from build123d import *

# Parameters (mm, degrees)
SKETCH_3_R               = 80
EXTRUDE_1_DEPTH          = 80
SKETCH_4_R               = 102.5
EXTRUDE_2_DEPTH          = 100
SKETCH_5_R               = 130
EXTRUDE_3_DEPTH          = 40
SKETCH_6_W               = 22
SKETCH_6_H               = 240.840734586
EXTRUDE_4_DEPTH          = 10
SHELL_START              = 82
SHELL_1_OUTLINE_R        = 100.5
SHELL_1_DEPTH            = 138
SHELL_START_2            = 2
SHELL_1_2_OUTLINE_R      = 78
SHELL_1_2_DEPTH          = 80
SHELL_START_3            = 182
SHELL_1_3_OUTLINE_R      = 128
SHELL_1_3_OUTLINE_R_2    = 100.5
SHELL_1_3_DEPTH          = 38
SHELL_START_4            = 212
SHELL_1_4_DEPTH          = 8
SKETCH_7_R               = 8.399329468
EXTRUDE_5_DEPTH          = 20
PATTERN_CIRCULAR_1_COUNT = 3
SKETCH_9_W               = 22
SKETCH_9_H               = 2
CUT_EXTRUDE_1_DEPTH      = 365.969552782
SKETCH_10_W              = 2
SKETCH_10_H              = 236.138085802
SKETCH_10_H_2            = 174.695606664
EXTRUDE_6_DEPTH          = 3
SKETCH_11_W              = 22
SKETCH_11_H              = 10
EXTRUDE_7_DEPTH          = 2
SKETCH_12_R              = 9.35670837
CUT_EXTRUDE_2_DEPTH      = 360.759328521
SKETCH_13_R              = 2.613319885
EXTRUDE_8_DEPTH          = 16
SKETCH_14_R              = 0.941183601
EXTRUDE_9_DEPTH          = 10


# Read off the part's stored shape, not the designer's step: 抽壳1
with BuildPart() as part:
    # 草图3 → 凸台-拉伸1 (new body)
    with BuildSketch(Plane(origin=(0, 0, 0), x_dir=(1, 0, 0), z_dir=(0, 1, 0))):
        with Locations(Location((0, 0, 0), (0, 0, 270))):
            Circle(SKETCH_3_R)
    extrude(amount=EXTRUDE_1_DEPTH)

    # 草图4 → 凸台-拉伸2 (add)
    with BuildSketch(Plane(origin=(0, 80, 0), x_dir=(1, 0, 0), z_dir=(0, 1, 0))):
        with Locations(Location((0, 0, 0), (0, 0, 270))):
            Circle(SKETCH_4_R)
    extrude(amount=EXTRUDE_2_DEPTH)

    # 草图5 → 凸台-拉伸3 (add)
    with BuildSketch(Plane(origin=(0, 180, 0), x_dir=(1, 0, 0), z_dir=(0, 1, 0))):
        with Locations(Location((0, 0, 0), (0, 0, 270))):
            Circle(SKETCH_5_R)
    extrude(amount=EXTRUDE_3_DEPTH)

    # 草图6 → 凸台-拉伸4 (add)
    with BuildSketch(Plane(origin=(0, 220, 0), x_dir=(1, 0, 0), z_dir=(0, 1, 0))):
        with Locations((117.8420905, -121.866187138)):
            Rectangle(SKETCH_6_W, SKETCH_6_H)
    extrude(amount=-EXTRUDE_4_DEPTH)

    # 抽壳1 outline → 抽壳1 (cut)
    with BuildSketch(Plane(origin=(0, 0, 0), x_dir=(1, 0, 0), z_dir=(0, 1, 0)).offset(SHELL_START)):
        Circle(SHELL_1_OUTLINE_R)
    extrude(amount=SHELL_1_DEPTH, mode=Mode.SUBTRACT)

    # Shell 1 2 outline → Shell 1 2 (cut)
    with BuildSketch(Plane(origin=(0, 0, 0), x_dir=(1, 0, 0), z_dir=(0, 1, 0)).offset(SHELL_START_2)):
        Circle(SHELL_1_2_OUTLINE_R)
    extrude(amount=SHELL_1_2_DEPTH, mode=Mode.SUBTRACT)

    # Shell 1 3 outline → Shell 1 3 (cut)
    with BuildSketch(Plane(origin=(0, 0, 0), x_dir=(1, 0, 0), z_dir=(0, 1, 0)).offset(SHELL_START_3)):
        Circle(SHELL_1_3_OUTLINE_R)
        Circle(SHELL_1_3_OUTLINE_R_2, mode=Mode.SUBTRACT)
    extrude(amount=SHELL_1_3_DEPTH, mode=Mode.SUBTRACT)

    # Shell 1 4 outline → Shell 1 4 (cut)
    with BuildSketch(Plane(origin=(0, 0, 0), x_dir=(1, 0, 0), z_dir=(0, 1, 0)).offset(SHELL_START_4)):
        with BuildLine():
            ThreePointArc((126.8420905, -17.178011456), (120.483699417, -43.216642337), (108.8420905, -67.360220721))
            Line((108.8420905, -67.360220721), (108.8420905, -240.286554431))
            Line((108.8420905, -240.286554431), (126.8420905, -240.286554431))
            Line((126.8420905, -240.286554431), (126.8420905, -17.178011456))
        make_face()
    extrude(amount=SHELL_1_4_DEPTH, mode=Mode.SUBTRACT)

    # 草图7 → 凸台-拉伸5 (add)
    with BuildSketch(Plane.XZ):
        with Locations(Location((0, 63.429571018, 0), (0, 0, 90))):
            Circle(SKETCH_7_R)
    extrude_5 = extrude(amount=EXTRUDE_5_DEPTH)

    # 阵列(圆周)1: 凸台-拉伸5 ×3 about axis
    pattern_circular_1_axis = Axis((0, 0, 0), (0, 1, 0))
    for i in range(1, PATTERN_CIRCULAR_1_COUNT):
        add(extrude_5.rotate(pattern_circular_1_axis, i * 360 / PATTERN_CIRCULAR_1_COUNT))

    # 草图9 → 切除-拉伸1 (cut, through all)
    with BuildSketch(Plane(origin=(0, 220, 0), x_dir=(1, 0, 0), z_dir=(0, 1, 0))):
        with Locations((117.8420905, -241.286554431)):
            Rectangle(SKETCH_9_W, SKETCH_9_H)
    extrude(amount=-CUT_EXTRUDE_1_DEPTH, mode=Mode.SUBTRACT)

    # 草图10 → 凸台-拉伸6 (add)
    with BuildSketch(Plane(origin=(0, 220, 0), x_dir=(1, 0, 0), z_dir=(0, 1, 0))):
        with Locations((109.8420905, -122.21751153)):
            Rectangle(SKETCH_10_W, SKETCH_10_H)
        with Locations((125.8420905, -152.938751099)):
            Rectangle(SKETCH_10_W, SKETCH_10_H_2)
    extrude(amount=-EXTRUDE_6_DEPTH)

    # 草图11 → 凸台-拉伸7 (add)
    with BuildSketch(Plane.XY.offset(240.286554431)):
        with Locations((117.8420905, 215)):
            Rectangle(SKETCH_11_W, SKETCH_11_H)
    extrude(amount=EXTRUDE_7_DEPTH)

    # 草图12 → 切除-拉伸2 (cut, through all)
    with BuildSketch(Plane(origin=(0, 212, 0), x_dir=(1, 0, 0), z_dir=(0, 1, 0))):
        with Locations(Location((117.8420905, -231.286554431, 0), (0, 0, 254.128345291))):
            Circle(SKETCH_12_R)
    extrude(amount=-CUT_EXTRUDE_2_DEPTH, mode=Mode.SUBTRACT)

    # 草图13 → 凸台-拉伸8 (add)
    with BuildSketch(Plane(origin=(128.8420905, 0, 0), x_dir=(0, 0, -1), z_dir=(1, 0, 0))):
        with Locations((-232.319143826, 214.997371462)):
            Circle(SKETCH_13_R)
    extrude(amount=EXTRUDE_8_DEPTH)

    # 草图14 → 凸台-拉伸9 (add)
    with BuildSketch(Plane(origin=(144.8420905, 0, 0), x_dir=(0, 0, -1), z_dir=(1, 0, 0))):
        with Locations((-232.319143826, 214.997371462)):
            Circle(SKETCH_14_R)
    extrude(amount=EXTRUDE_9_DEPTH)


solid = part.part
CAD build for the part. Positions are in the model's coordinates, mm. A direction names the side the tool comes from. Round coordinates to 2 decimals unless told otherwise and drop trailing zeros. Write each loop counter-clockwise with the first axis right and the second up, starting at its lowest first coordinate (ties: lowest second). Pieces come first, ordered by that corner, then holes.
(1) Slice it at D-D, the plane z = -50. Write the cut outline in (x, y), and give its area (3 significant figures).
(2) Slice it at A-A, the plane z = 153.5. Write the cut outline in (x, y).
(3) Probe line 1 along X through (y, z) = (210, 0); line 2 along X through (y, z) = (25, 0). List the from-to ranges inside material, lowest first.
(4) Slice it at C-C, the plane y = 26. Write the cut outline in (x, z).
(5) 3-axis set-ups, long thin cutter, end or side, ignore diameter. For faces 1 (the face through (118, 216, 240.287)), 2 (the face through (-10.154, 41.44, -77.336)), 3 (the face through (118, 210, 128)), 4 (the face through (39, 180, 96)): which of +Z, -Z, +X, -X, +Y, -Y reach the whole face in a straight line?
(6) Slice it at B-B, the plane x = 0. Write the cut outline in (y, z), and give its area (3 significant figures).
(7) Drop flat-ended pins along their axis: P1, Ø12, axis at x = 64, y = 194.5, coming from the +Z side; P2, Ø2, axis at x = 110, z = 121, coming from the -Y side; P3, Ø3, axis at x = -80.5, y = 107, coming from the +Z side. Give the stop position or say it passes through.
(8) Mould opens along X. For faces 5 (the face through (55, -20, -32)), 6 (the face through (126.842, 215, 130)), 7 (the face through (-78.1, 39.44, -17.34)) say: pulls with the +X half, pulls with the -X half, needs draft (parallel to the pull), parting line crosses it, or undercut.
From the geometry:
1. outline: (-120, 180) - (-89.48, 180) - (-89.48, 80) - (-62.45, 80) - (-62.45, 0) - (62.45, 0) - (62.45, 80) - (89.48, 80) - (89.48, 180) - (120, 180) - (120, 220) - (117.83, 220) - (117.83, 182) - (87.18, 182) - (87.18, 82) - (59.87, 82) - (59.87, 2) - (-59.87, 2) - (-59.87, 82) - (-87.18, 82) - (-87.18, 182) - (-117.83, 182) - (-117.83, 220) - (-120, 220) - close
1. area: 1,520 mm2
2. outline: (106.84, 210) - (128.84, 210) - (128.84, 220) - (124.84, 220) - (124.84, 217) - (126.84, 217) - (126.84, 212) - (108.84, 212) - (108.84, 217) - (110.84, 217) - (110.84, 220) - (106.84, 220) - close
3. line 1: x = -130 to -128, 128 to 130
3. line 2: x = -80 to -78, 78 to 80
4. outline: circle Ø160 at (0, 0); hole circle Ø156 at (0, 0)
5. face 1: none
5. face 2: +Y
5. face 3: +Z, +X, -Y
5. face 4: -Y
6. outline: (-20, 55.03) - (0, 55.03) - (0, -80) - (80, -80) - (80, -102.5) - (180, -102.5) - (180, -130) - (220, -130) - (220, -128) - (182, -128) - (182, -100.5) - (82, -100.5) - (82, -78) - (2, -78) - (2, 78) - (82, 78) - (82, 100.5) - (182, 100.5) - (182, 128) - (220, 128) - (220, 130) - (180, 130) - (180, 102.5) - (80, 102.5) - (80, 80) - (0, 80) - (0, 71.83) - (-20, 71.83) - close
6. area: 1,730 mm2
7. P1: stops at z = 116.34
7. P2: stops at y = 210
7. P3: stops at z = 65.31
8. face 5: needs draft
8. face 6: undercut
8. face 7: parting line crosses it
